```python
from build123d import *

# Parameters (mm, degrees)
ESQUISSE1_R                  = 3
BASE_EXTRUSION_DEPTH         = 15
ESQUISSE2_R                  = 4.5
BOSS_EXTRU_1_DEPTH           = 5
ENL_V_MAT_EXTRU_3_DEPTH      = 4
R_P_TITION_CIRCULAIRE1_COUNT = 6


with BuildPart() as part:
    # Esquisse1 → Base-Extrusion (new body)
    with BuildSketch(Plane.XY):
        Circle(ESQUISSE1_R)
    extrude(amount=BASE_EXTRUSION_DEPTH)

    # Esquisse2 → Boss.-Extru.1 (add)
    with BuildSketch(Plane(origin=(0, 0, 0), x_dir=(-1, 0, 0), z_dir=(0, 0, -1))):
        Circle(ESQUISSE2_R)
    extrude(amount=BOSS_EXTRU_1_DEPTH)

    # Esquisse3 → Enlèv. mat.-Extru.3 (cut)
    with BuildSketch(Plane(origin=(0, 0, -5), x_dir=(-1, 0, 0), z_dir=(0, 0, -1))):
        Polygon((3, 1.732050808), (0, 0), (3, -1.732050808), align=None)
    enl_v_mat_extru_3 = extrude(amount=-ENL_V_MAT_EXTRU_3_DEPTH, mode=Mode.SUBTRACT)

    # Répétition circulaire1: Enlèv. mat.-Extru.3 ×6 about axis
    r_p_tition_circulaire1_axis = Axis((0, 0, 0), (0, 0, 1))
    for i in range(1, R_P_TITION_CIRCULAIRE1_COUNT):
        add(enl_v_mat_extru_3.rotate(r_p_tition_circulaire1_axis, i * 360 / R_P_TITION_CIRCULAIRE1_COUNT), mode=Mode.SUBTRACT)


solid = part.part
```
Model file for the job. Use its own axes, mm. A direction names the side the tool comes from. Coordinates: 2 decimals unless noted, no trailing zeros. Order: outer loops, then holes, each group sorted by start corner. A loop starts at its lowest first (then second) coordinate and runs counter-clockwise, first axis right, second up. Notation, with made-up numbers: (-15, -4.5) -> (29, -4.5) arc R34 ccw to (29, 25.5) -> close; hole circle Ø10 at (41, 49.25). An arc over 180 degrees is marked (long way). Return JSON: item names as keys, results as strings.
Item 1: Slice it at C-C (z = 0.25). Write the cut outline in (x, y), then the cut area to 3 significant figures.
Model answer:
{"outline": "circle Ø6 at (0, 0)", "area": "28.3 mm²"}
Item 2: Slice it at A-A (y = 0). Write the cut outline in (x, z).
Model answer:
{"outline": "(-4.5, -5) -> (-3, -5) -> (-3, -1) -> (3, -1) -> (3, -5) -> (4.5, -5) -> (4.5, 0) -> (3, 0) -> (3, 15) -> (-3, 15) -> (-3, 0) -> (-4.5, 0) -> close"}
Item 3: Slice it at B-B (x = 1.5). Write the cut outline in (y, z).
Model answer:
{"outline": "(-4.24, -5) -> (-2.6, -5) -> (-2.6, -1) -> (2.6, -1) -> (2.6, -5) -> (4.24, -5) -> (4.24, 0) -> (2.6, 0) -> (2.6, 15) -> (-2.6, 15) -> (-2.6, 0) -> (-4.24, 0) -> close"}
Item 4: Mould opens along X. For faces 1 (the face through (3, 0, -3)), 2 (the face through (1.5, -2.6, -3)), 3 (the face through (0.59, 4.46, -2.46)), 4 (the face through (1.1, 3.1, -5)) say: pulls with the +X half, pulls with the -X half, needs draft (parallel to the pull), parting line crosses it, or undercut.
Model answer:
{"face 1": "undercut", "face 2": "undercut", "face 3": "parting line crosses it", "face 4": "needs draft"}
Item 5: Pin check, flat tips, straight feed: P1, Ø3, axis at x = 2.5, z = 8.5, coming from the -Y side; P2, Ø1.8, axis at x = -1, y = -1, coming from the -Z side; P3, Ø1.5, axis at x = -3, y = -2.5, coming from the +Z side. Stop position of each tip, or through.
Model answer:
{"P1": "stops at y = -2.83", "P2": "stops at z = -1", "P3": "stops at z = 0"}
Item 6: Wall check: line 1 along Z through (x, y) = (-2, 0.5); line 2 along X through (y, z) = (-0.5, -2); line 3 along Z through (x, y) = (2.5, 2.5). Give the ranges that are in metal, low to high. Write a range as from..to.
Model answer:
{"line 1": "z = -1..15", "line 2": "x = -4.47..-3, 3..4.47", "line 3": "z = -5..0"}
Item 7: 3-axis set-ups, long thin cutter, end or side, ignore diameter. For faces 5 (the face through (0, 0, 15)), 6 (the face through (-3, 0, 7)), 7 (the face through (1.5, 2.6, -3)): which of +Z, -Z, +X, -X, +Y, -Y reach the whole face in a straight line?
Model answer:
{"face 5": "+Z, +X, -X, +Y, -Y", "face 6": "+Z", "face 7": "-Z"}
